CAD build for the part. Positions are in the model's coordinates, mm. Face numbers are marked on the shaded views. Give positions to 0.01 mm unless a question says otherwise; leave off trailing zeros. Loops run counter-clockwise (first coordinate to the right, second up) from the corner with the lowest first, then second, coordinate; pieces in that order, holes last.
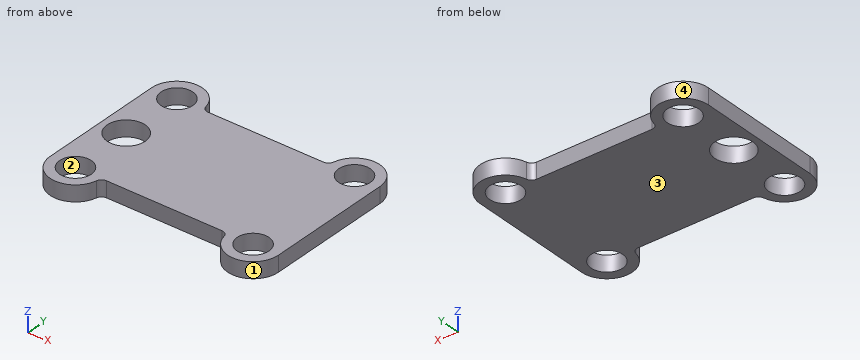
```python
from build123d import *

# Parameters (mm, degrees)
F0_R     = 30
F0_R_2   = 25
F1_DEPTH = 25
F2_R     = 10


with BuildPart() as f1:
    # F0 (on Top) → F1 (new body)
    with BuildSketch(Plane.XY):
        with BuildLine():
            Line((100, 100), (-100, 100))
            ThreePointArc((-100, 100), (-140, 60), (-180, 100))
            Line((-180, 100), (-180, -100))
            ThreePointArc((-180, -100), (-140, -60), (-100, -100))
            Line((-100, -100), (100, -100))
            ThreePointArc((100, -100), (140, -60), (180, -100))
            Line((180, -100), (180, 100))
            ThreePointArc((180, 100), (140, 60), (100, 100))
        make_face()
        with Locations((-140, 0)):
            Circle(F0_R, mode=Mode.SUBTRACT)
        with BuildLine():
            ThreePointArc((-180, 100), (-140, 60), (-100, 100))
            ThreePointArc((-100, 100), (-140, 140), (-180, 100))
        make_face()
        with Locations((-140, 100)):
            Circle(F0_R_2, mode=Mode.SUBTRACT)
        with BuildLine():
            ThreePointArc((180, 100), (140, 140), (100, 100))
            ThreePointArc((100, 100), (140, 60), (180, 100))
        make_face()
        with Locations((140, 100)):
            Circle(F0_R_2, mode=Mode.SUBTRACT)
        with BuildLine():
            ThreePointArc((100, -100), (140, -140), (180, -100))
            ThreePointArc((180, -100), (140, -60), (100, -100))
        make_face()
        with Locations((140, -100)):
            Circle(F0_R_2, mode=Mode.SUBTRACT)
        with BuildLine():
            ThreePointArc((-100, -100), (-140, -60), (-180, -100))
            ThreePointArc((-180, -100), (-140, -140), (-100, -100))
        make_face()
        with Locations((-140, -100)):
            Circle(F0_R_2, mode=Mode.SUBTRACT)
    extrude(amount=F1_DEPTH)

    # F2
    f2_edges = [f1.edges().sort_by_distance(p)[0] for p in [
        (-100, -100, 12.5),
        (100, -100, 12.5),
        (-100, 100, 12.5),
        (100, 100, 12.5),
    ]]
    fillet(f2_edges, radius=F2_R)


solid = f1.part
```
1. Probe line 1 along Y through (x, z) = (-140, 8.5); line 2 along Y through (x, z) = (-88, 17); line 3 along X through (y, z) = (92, 9.5). List the from-to ranges inside material, lowest first.
Responses:
line 1: y = -140 to -125, -75 to -30, 30 to 75, 125 to 140
line 2: y = -100 to 100
line 3: x = -180 to -163.69, -116.31 to 116.31, 163.69 to 180
2. Pull direction Y, two halves, no side cores. Call the marked faces 1, 2, 3 and 4: released by +Y, released by -Y, zero draft, split by the parting line, or undercut.
Responses:
face 1: released by -Y
face 2: undercut
face 3: zero draft
face 4: released by +Y
3. Saw through at A-A, the plane x = 140. List the corners of the cut face in (y, z), and give its area (3 significant figures).
Responses:
outline: (-140, 0) - (-125, 0) - (-125, 25) - (-140, 25) - close; (-75, 0) - (75, 0) - (75, 25) - (-75, 25) - close; (125, 0) - (140, 0) - (140, 25) - (125, 25) - close
area: 4,500 mm2
4. Saw through at C-C, the plane z = 4.75. List the corners of the cut face in (x, y), and give its area (3 significant figures).
Responses:
outline: (-180, -100) arc R40 ccw to (-100.81, -108) arc R10 cw to (-91.01, -100) - (91.01, -100) arc R10 cw to (100.81, -108) arc R40 ccw to (180, -100) - (180, 100) arc R40 ccw to (100.81, 108) arc R10 cw to (91.01, 100) - (-91.01, 100) arc R10 cw to (-100.81, 108) arc R40 ccw to (-180, 100) - close; hole circle Ø60 at (-140, 0); hole circle Ø50 at (-140, -100); hole circle Ø50 at (-140, 100); hole circle Ø50 at (140, -100); hole circle Ø50 at (140, 100)
area: 71,400 mm2
5. Saw through at B-B, the plane y = 0. List the corners of the cut face in (x, z).
Responses:
outline: (-180, 0) - (-170, 0) - (-170, 25) - (-180, 25) - close; (-110, 0) - (180, 0) - (180, 25) - (-110, 25) - close
6. Saw through at D-D, the plane x = -140. List the corners of the cut face in (y, z).
Responses:
outline: (-140, 0) - (-125, 0) - (-125, 25) - (-140, 25) - close; (-75, 0) - (-30, 0) - (-30, 25) - (-75, 25) - close; (30, 0) - (75, 0) - (75, 25) - (30, 25) - close; (125, 0) - (140, 0) - (140, 25) - (125, 25) - close
7. Drop flat-ended pins along their axis: pin 1 (12 mm diameter, centred on y = 104, z = 20.5, fed in from -X); pin 2 (12.5 mm diameter, centred on x = -23.5, z = 14.5, fed in from +Y); pin 3 (12.5 mm diameter, centred on x = -17, z = 13.5, fed in from -Y). Give the stop position or say it passes through.
Responses:
pin 1: stops at x = -180
pin 2: stops at y = 100
pin 3: stops at y = -100
